Drawing for the job (mm, zero at the part's lowest x, y, z). A direction names the side the tool comes from. Give positions to 0.01 mm unless a question says otherwise; leave off trailing zeros. Loops run counter-clockwise (first coordinate to the right, second up) from the corner with the lowest first, then second, coordinate; pieces in that order, holes last. Notation, with made-up numbers: (9, 82) -> (13, 82) arc R11 cw to (13, 91) -> close; hole circle Ø8 at (-14.5, -25). An arc over 180 degrees is marked (long way). Use CSV: the item, a comma, the result in double quotes. Start each with the question number.
(1) Flat gauge pins, fed straight in: pin 1 (9.5 mm diameter, centred on x = 51.5, y = 15.5, fed in from +Z); pin 2 (6.5 mm diameter, centred on x = 43, y = 6, fed in from +Z). Where does each tip first touch, or does it go through?
(2) Drill centre lines: probe 1 along Y at (x, z) = (42.5, 2); probe 2 along Y at (x, z) = (54, 1.25); probe 3 along X at (y, z) = (14.75, 3.75). Where is each one in solid material? Low to high.
(3) Cut at C-C on x = 34.5. Write the cut outline in (y, z), then the cut area to 4 significant figures.
(4) Cut at B-B on y = 20.25. Write the cut outline in (x, z), then the cut area to 3 significant figures.
(5) 3-axis set-ups, long thin cutter, end or side, ignore diameter. For the marked faces 1, 2 and 3: which of +Z, -Z, +X, -X, +Y, -Y reach the whole face in a straight line?
(6) Cut at A-A on z = 6. Write the cut outline in (x, y).
(7) Cut at D-D on z = 3.25. Write the cut outline in (x, y), then the cut area to 4 significant figures.
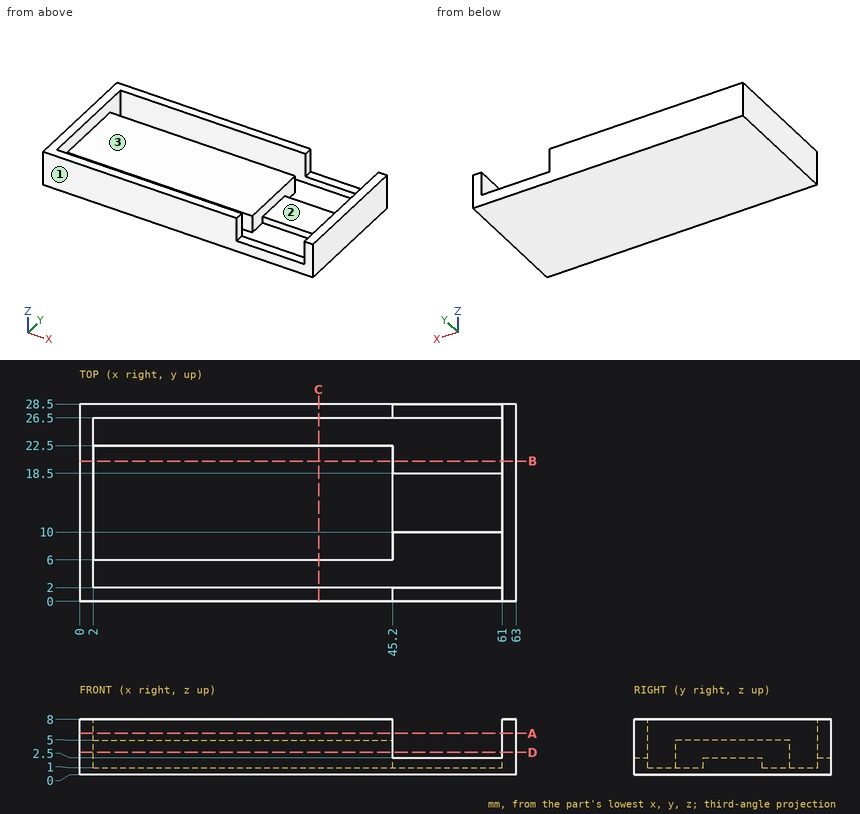
Check result:
1,pin 1,"z = 2.5"
1,pin 2,"z = 5"
2,probe 1,"0 to 2, 6 to 22.5, 26.5 to 28.5"
2,probe 2,"0 to 2, 10 to 18.5, 26.5 to 28.5"
2,probe 3,"0 to 45.2, 61 to 63"
3,outline,"(0, 0) -> (28.5, 0) -> (28.5, 8) -> (26.5, 8) -> (26.5, 1) -> (22.5, 1) -> (22.5, 5) -> (6, 5) -> (6, 1) -> (2, 1) -> (2, 8) -> (0, 8) -> close"
3,area,"122.5 mm²"
4,outline,"(0, 0) -> (63, 0) -> (63, 8) -> (61, 8) -> (61, 1) -> (45.2, 1) -> (45.2, 5) -> (2, 5) -> (2, 8) -> (0, 8) -> close"
4,area,"264 mm²"
5,face 1,"+Z, -Z, +X, -X, -Y"
5,face 2,"+Z, +Y, -Y"
5,face 3,"+Z"
6,outline,"(0, 0) -> (45.2, 0) -> (45.2, 2) -> (2, 2) -> (2, 26.5) -> (45.2, 26.5) -> (45.2, 28.5) -> (0, 28.5) -> close; (61, 0) -> (63, 0) -> (63, 28.5) -> (61, 28.5) -> close"
7,outline,"(0, 0) -> (45.2, 0) -> (45.2, 2) -> (2, 2) -> (2, 6) -> (45.2, 6) -> (45.2, 22.5) -> (2, 22.5) -> (2, 26.5) -> (45.2, 26.5) -> (45.2, 28.5) -> (0, 28.5) -> close; (61, 0) -> (63, 0) -> (63, 28.5) -> (61, 28.5) -> close"
7,area,"1,000 mm²"
